Part model, mm, in its own coordinate system. A direction names the side the tool comes from. Coordinates: 2 decimals unless noted, no trailing zeros. Loops run counter-clockwise (first coordinate to the right, second up) from the corner with the lowest first, then second, coordinate; pieces in that order, holes last. Notation, with made-up numbers: (2.5, 3.5) -> (49.5, 3.5) arc R16 cw to (49.5, 21.5) -> close; hole circle Ø6 at (68, -21.75). An arc over 180 degrees is marked (long way). One line per question, with ' | ' between items. Start each with the question number.
1) Probe L1, parallel to Y at x = 5.75, z = 2.5; L2, parallel to X at y = -7, z = 0.25; L3, parallel to Z at x = 3, y = 35. List the from-to ranges inside material, lowest first. Write a range as from..to.
2) Two-plate mould, pull along Y, no slides. Class faces 5 (the face through (9.76, -0.16, -2.17)), 6 (the face through (-8.43, 11.76, 4.38)), 7 (the face through (10, -11.1, 3)), 8 (the face through (0, -42.5, 0)): released by +Y, released by -Y, zero draft, split by the parting line, or undercut.
3) Drop flat-ended pins along their axis: pin 1 (6 mm diameter, centred on x = -9, y = 24.5, fed in from -Z); pin 2 (3 mm diameter, centred on x = 1, y = 3.5, fed in from -Z); pin 3 (10 mm diameter, centred on y = -31, z = -3.5, fed in from -X). Give the stop position or say it passes through.
4) Cut at D-D (y = 37.5). List the corners of the cut face in (x, z).
5) Cut at C-C (y = -20). List the corners of the cut face in (x, z), plus the area to 3 significant figures.
6) 3-axis set-ups, long thin cutter, end or side, ignore diameter. For faces 1 (the face through (-4, 12.4, 9)), 2 (the face through (4.88, 34.4, -1.08)), 3 (the face through (4.88, -34.6, -1.08)), 4 (the face through (-4.43, -19.15, 14.07)): which of +Z, -Z, +X, -X, +Y, -Y reach the whole face in a straight line?
Autodesk Inventor part; units mm, degrees
ref_plane "YZ Plane" through (0, 0, 0) normal (1, 0, 0) x (0, 1, 0)
ref_plane "XZ Plane" through (0, 0, 0) normal (0, 1, 0) x (-1, 0, 0)
ref_plane "XY Plane" through (0, 0, 0) normal (0, 0, 1) x (1, 0, 0)
sketch "Skizze1" plane through (0, 0, 0) normal (1, 0, 0) x (0, 1, 0)
  line L0 (0, 17.7) -> (0, -2.95) construction
  line L1 (-59.5, 0) -> (59.5, 0)
  line L2 (42.5, 5) -> (42.5, 0)
  line L3 (42.5, 5) -> (27.5, 5)
  line L4 (27.5, 5) -> (27.5, 10)
  line L5 (27.5, 10) -> (-11.1, 10)
  line L6 (-11.1, 10) -> (-11.1, 14.75)
  line L7 (-11.1, 14.75) -> (-27.5, 14.75)
  line L8 (-27.5, 14.75) -> (-27.5, 5)
  line L9 (-27.5, 5) -> (-42.5, 5)
  line L10 (-42.5, 5) -> (-42.5, 0)
  line L11 (-11.1, 14.75) -> (11.1, 14.75) construction
  line L12 (11.1, 14.75) -> (11.1, 10) construction
  line L13 (-42.5, 0) -> (42.5, 0)
  point P0 (0, 0)
  dimension "d0" = 10
  dimension "d1" = 15
  dimension "d2" = 22.2
  dimension "d3" = 55
  dimension "d4" = 20
  dimension "d5" = 29.5
revolve "Grundkörper" add sketch "Skizze1" angle 360 about axis through (0, 0, 0) along (0, 1, 0)
sketch "Skizze2" plane through (0, 0, 0) normal (1, 0, 0) x (0, 1, 0)
  line L0 (-18.82, 0) -> (35.22, 0) construction
  line L1 (-11.1, -14.75) -> (-11.1, 14.75) construction
  line L2 (-11.1, 10) -> (27.5, 10)
  line L3 (-11.1, 10) -> (-11.1, 14.75)
  line L4 (-11.1, 14.75) -> (11.1, 14.75)
  line L5 (11.1, 14.75) -> (11.1, 10)
  line L6 (11.1, 10) -> (-11.1, 10)
  line L7 (0, 20.65) -> (0, -20.65) construction
  line L8 (11.1, 10) -> (11.1, 9.5)
  line L9 (11.1, 9.5) -> (12.4, 9.5)
  line L10 (12.4, 9.5) -> (12.4, 10)
  line L11 (11.1, 10) -> (12.4, 10)
  point P0 (0, 0)
  dimension "d15" = 1.3
  dimension "d16" = 19
revolve "Nut_Sicherungsring_DIN471-20x1,2" cut sketch "Skizze2" angle 360 about axis through (0, 0, 0) along (0, 1, 0) contours L2 L10 L9 L8
chamfer "FaseAllgemein" distance 1 angle 45 3 edges at (0, -42.5, -5) (0, 42.5, -5) (0, -27.5, -14.75)
chamfer "FaseLager" distance 0.5 angle 45 1 edges at (0, -11.1, -14.75)
properties part number "200-40-BOGIE-CONNECTOR-05" material "Aluminium 6061"
Reported:
1) L1: y = -27.5..27.5 | L2: x = -10..10 | L3: z = -4..4
2) face 5: zero draft | face 6: undercut | face 7: released by +Y | face 8: released by -Y
3) pin 1: stops at z = -8 | pin 2: stops at z = -10 | pin 3: stops at x = -14.69
4) outline: circle Ø10 at (0, 0)
5) outline: circle Ø29.5 at (0, 0) | area: 683 mm²
6) face 1: none | face 2: +Y | face 3: -Y | face 4: +Y, -Y
